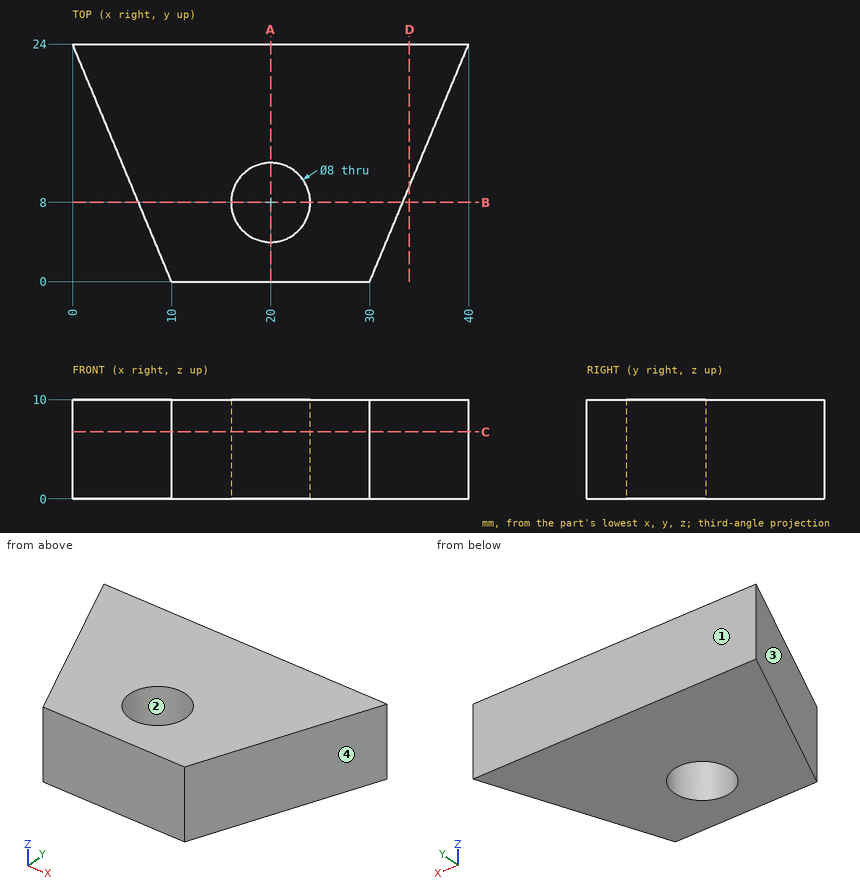
Design review of the part shown in the three views and the two pictorial views. Dimensions are in mm from the part's minimum x, y and z. Round coordinates to 2 decimals unless told otherwise and drop trailing zeros. Write each loop counter-clockwise with the first axis right and the second up, starting at its lowest first coordinate (ties: lowest second). Pieces come first, ordered by that corner, then holes.
Item 1: We need section D-D on x = 34. Write out the cut boundary in (y, z), and give its area (3 significant figures).
Item 2: We need section B-B on y = 8. Write out the cut boundary in (x, z).
Item 3: The part is to be moulded in two halves that separate along X. For the marked faces 1, 2, 3 and 4, say which applies: +X half, -X half, draft (parallel to the pull), parting line (faces both ways), or undercut.
Item 4: For probe 1 along Y at (x, z) = (20, 5.75); probe 2 along X at (y, z) = (10, 7); probe 3 along X at (y, z) = (10.5, 1) (1 decimal), list the stretches that pass through material, from the lowest coordinate up.
Item 5: We need section C-C on z = 6.75. Write out the cut boundary in (x, y), and give its area (3 significant figures).
Item 6: We need section A-A on x = 20. Write out the cut boundary in (y, z), and give its area (3 significant figures).
Item 7: Clearance check with flat-ended pins moving along their axes: pin 1 Ø5 at (y, z) = (13, 4.5) entering from +X; pin 2 Ø1 at (y, z) = (11, 2.5) entering from +X; pin 3 Ø2 at (y, z) = (19.5, 4) entering from -X. State where each tip first meets the part, or that it passes through.
Returned:
1. outline: (9.6, 0) - (24, 0) - (24, 10) - (9.6, 10) - close
1. area: 144 mm2
2. outline: (6.67, 0) - (16, 0) - (16, 10) - (6.67, 10) - close; (24, 0) - (33.33, 0) - (33.33, 10) - (24, 10) - close
3. face 1: draft
3. face 2: undercut
3. face 3: -X half
3. face 4: +X half
4. probe 1: y = 0 to 4, 12 to 24
4. probe 2: x = 5.83 to 16.54, 23.46 to 34.17
4. probe 3: x = 5.6 to 16.9, 23.1 to 34.4
5. outline: (0, 24) - (10, 0) - (30, 0) - (40, 24) - close; hole circle Ø8 at (20, 8)
5. area: 670 mm2
6. outline: (0, 0) - (4, 0) - (4, 10) - (0, 10) - close; (12, 0) - (24, 0) - (24, 10) - (12, 10) - close
6. area: 160 mm2
7. pin 1: stops at x = 36.46
7. pin 2: stops at x = 34.79
7. pin 3: stops at x = 1.46
